```python
from build123d import *
from OCP.BRepAlgoAPI import BRepAlgoAPI_Cut
from OCP.TopTools import TopTools_ListOfShape

# Parameters (mm, degrees)
SKETCH3_R                = 3.65
SKETCH3_R_2              = 2.1
BOSS_EXTRUDE3_DEPTH      = 15
BOSS_EXTRUDE4_DEPTH      = 8
BOSS_EXTRUDE4_DEPTH_BACK = 8
SKETCH7_R                = 2.1
CUT_EXTRUDE1_DEPTH       = 18
FILLET2_START            = -8
FILLET2_DEPTH            = 16
FILLET2_2_ANGLE          = 28.578113
FILLET2_3_ANGLE          = 28.578113


with BuildPart() as part:
    # Sketch3 → Boss-Extrude3 (new body)
    with BuildSketch(Plane(origin=(0, 0, 0), x_dir=(0, 0, -1), z_dir=(1, 0, 0))):
        Circle(SKETCH3_R)
        Circle(SKETCH3_R_2, mode=Mode.SUBTRACT)
    extrude(amount=BOSS_EXTRUDE3_DEPTH)

    # Sketch6 → Boss-Extrude4 (add, two sides: drawn at the far end of the back side and taken through both)
    with BuildSketch(Plane(origin=(0, 0, 0), x_dir=(1, 0, 0), z_dir=(0, 1, 0)).offset(-BOSS_EXTRUDE4_DEPTH_BACK)):
        with BuildLine():
            Line((3.477507, 8.380826), (4.919958, 8.978308))
            ThreePointArc((4.919958, 8.978308), (6.258182, -0.050001), (5.26999, -9.123296))
            Line((5.26999, -9.123296), (3.819467, -8.52247))
            ThreePointArc((3.819467, -8.52247), (4.707866, -0.049391), (3.477507, 8.380826))
        make_face()
    extrude(amount=BOSS_EXTRUDE4_DEPTH + BOSS_EXTRUDE4_DEPTH_BACK)

    # Sketch7 → Cut-Extrude1 (cut)
    with BuildSketch(Plane.ZY):
        with Locations(Location((0, 0, 0), (0, 0, 180))):
            Circle(SKETCH7_R)
    extrude(amount=-CUT_EXTRUDE1_DEPTH, mode=Mode.SUBTRACT)


with BuildPart() as fillet2_tool:
    # Fillet2: read off the stored shape, not the designer's step
    # Fillet2 outline → Fillet2 (new body)
    with BuildSketch(Plane(origin=(0, 0, 0), x_dir=(1, 0, 0), z_dir=(0, 1, 0)).offset(FILLET2_START)):
        with BuildLine():
            ThreePointArc((5.26999, -9.123296), (5.521856, -7.99803), (5.737351, -6.865235))
            ThreePointArc((5.737351, -6.865235), (5.074459, -8.036465), (3.819467, -8.52247))
            Line((3.819467, -8.52247), (5.26999, -9.123296))
        make_face()
        with BuildLine():
            ThreePointArc((3.477507, 8.380826), (4.751128, 7.945976), (5.460847, 6.802514))
            ThreePointArc((5.460847, 6.802514), (5.20744, 7.894646), (4.919958, 8.978308))
            Line((4.919958, 8.978308), (3.477507, 8.380826))
        make_face()
    extrude(amount=FILLET2_DEPTH)


with BuildPart() as part_1:
    add(part.part)

    # Fillet2: cut by fillet2_tool, with a tolerance
    fillet2_stock = TopTools_ListOfShape()
    fillet2_stock.Append(part_1.part.wrapped)
    fillet2_tools = TopTools_ListOfShape()
    fillet2_tools.Append(fillet2_tool.part.wrapped)
    fillet2_cut = BRepAlgoAPI_Cut()
    fillet2_cut.SetArguments(fillet2_stock)
    fillet2_cut.SetTools(fillet2_tools)
    fillet2_cut.SetFuzzyValue(0.00001)
    fillet2_cut.Build()
    add(Compound.cast(fillet2_cut.Shape()).solids(), mode=Mode.REPLACE)


with BuildPart() as fillet2_2_tool:
    # Fillet2 2 outline → Fillet2 2 (revolve)
    with BuildSketch(Plane(origin=(-29.535127, 0, 0.742139), x_dir=(0.9738567621765157, 0, 0.22716295200378364), z_dir=(-0.22716295200378364, 0, 0.9738567621765157))):
        with BuildLine():
            Line((35.8, -8), (35.8, -6.051282))
            ThreePointArc((35.8, -6.051282), (35.365248, -7.296272), (34.25, -8))
            Line((34.25, -8), (35.8, -8))
        make_face()
    revolve(axis=Axis((-29.535127, 0, 0.742139), (0, 1, 0)), revolution_arc=FILLET2_2_ANGLE)


with BuildPart() as part_2:
    add(part_1.part)

    # Fillet2 2: cut by fillet2_2_tool, with a tolerance
    fillet2_2_stock = TopTools_ListOfShape()
    fillet2_2_stock.Append(part_2.part.wrapped)
    fillet2_2_tools = TopTools_ListOfShape()
    fillet2_2_tools.Append(fillet2_2_tool.part.wrapped)
    fillet2_2_cut = BRepAlgoAPI_Cut()
    fillet2_2_cut.SetArguments(fillet2_2_stock)
    fillet2_2_cut.SetTools(fillet2_2_tools)
    fillet2_2_cut.SetFuzzyValue(0.00001)
    fillet2_2_cut.Build()
    add(Compound.cast(fillet2_2_cut.Shape()).solids(), mode=Mode.REPLACE)


with BuildPart() as fillet2_3_tool:
    # Fillet2 3 outline → Fillet2 3 (revolve)
    with BuildSketch(Plane(origin=(-29.535127, 0, 0.742139), x_dir=(0.9738567621765157, 0, 0.22716295200378342), z_dir=(-0.22716295200378342, 0, 0.9738567621765157))):
        with BuildLine():
            ThreePointArc((34.25, 8), (35.365248, 7.296272), (35.8, 6.051282))
            Line((35.8, 6.051282), (35.8, 8))
            Line((35.8, 8), (34.25, 8))
        make_face()
    revolve(axis=Axis((-29.535127, 0, 0.742139), (0, 1, 0)), revolution_arc=FILLET2_3_ANGLE)


with BuildPart() as part_3:
    add(part_2.part)

    # Fillet2 3: cut by fillet2_3_tool, with a tolerance
    fillet2_3_stock = TopTools_ListOfShape()
    fillet2_3_stock.Append(part_3.part.wrapped)
    fillet2_3_tools = TopTools_ListOfShape()
    fillet2_3_tools.Append(fillet2_3_tool.part.wrapped)
    fillet2_3_cut = BRepAlgoAPI_Cut()
    fillet2_3_cut.SetArguments(fillet2_3_stock)
    fillet2_3_cut.SetTools(fillet2_3_tools)
    fillet2_3_cut.SetFuzzyValue(0.00001)
    fillet2_3_cut.Build()
    add(Compound.cast(fillet2_3_cut.Shape()).solids(), mode=Mode.REPLACE)


solid = part_3.part
```
Build history of the part. All positions in model axes, mm. A direction names the side the tool comes from. Coordinates: 2 decimals unless noted, no trailing zeros. Order: outer loops, then holes, each group sorted by start corner. A loop starts at its lowest first (then second) coordinate and runs counter-clockwise, first axis right, second up.
Item 1: Saw through at C-C on y = -2.5. List the corners of the cut face in (x, z), then the cut area to 3 significant figures.
Filled in:
outline: (0, -2.66) - (4.55, -2.66) arc R34.25 cw to (3.48, -8.38) arc R2 ccw to (5.46, -6.8) arc R35.8 ccw to (6.1, -2.66) - (15, -2.66) - (15, 2.66) - (6.21, 2.66) arc R35.8 ccw to (5.74, 6.87) arc R2 ccw to (3.82, 8.52) arc R34.25 cw to (4.66, 2.66) - (0, 2.66) - close
area: 97.0 mm2
Item 2: Drop flat-ended pins along their axis: pin 1 Ø1 at (x, z) = (13.5, 6) entering from -Y; pin 2 Ø1 at (x, z) = (3.5, -2) entering from -Y; pin 3 Ø1.5 at (x, y) = (8, -2) entering from +Z; pin 4 Ø8 at (x, z) = (8.5, -4) entering from -Y. Give the stop position or say it passes through.
Filled in:
pin 1: passes through
pin 2: stops at y = -3.33
pin 3: stops at z = 3.43
pin 4: stops at y = -7.98
Item 3: Saw through at A-A on y = 0. List the corners of the cut face in (x, z).
Filled in:
outline: (0, -3.65) - (4.43, -3.65) arc R34.25 cw to (3.48, -8.38) arc R2 ccw to (5.46, -6.8) arc R35.8 ccw to (5.99, -3.65) - (15, -3.65) - (15, -2.1) - (0, -2.1) - close; (0, 2.1) - (15, 2.1) - (15, 3.65) - (6.15, 3.65) arc R35.8 ccw to (5.74, 6.87) arc R2 ccw to (3.82, 8.52) arc R34.25 cw to (4.59, 3.65) - (0, 3.65) - close
Item 4: Saw through at B-B on x = 11. List the corners of the cut face in (y, z), then the cut area to 3 significant figures.
Filled in:
outline: circle Ø7.3 at (0, 0); hole circle Ø4.2 at (0, 0)
area: 28.0 mm2
Item 5: Saw through at D-D on y = 1.75. List the corners of the cut face in (x, z), then the cut area to 3 significant figures.
Filled in:
outline: (0, -3.2) - (4.49, -3.2) arc R34.25 cw to (3.48, -8.38) arc R2 ccw to (5.46, -6.8) arc R35.8 ccw to (6.05, -3.2) - (15, -3.2) - (15, -1.16) - (0, -1.16) - close; (0, 1.16) - (15, 1.16) - (15, 3.2) - (6.18, 3.2) arc R35.8 ccw to (5.74, 6.87) arc R2 ccw to (3.82, 8.52) arc R34.25 cw to (4.63, 3.2) - (0, 3.2) - close
area: 76.8 mm2
Item 6: Tool access for faces 1 (the cylindrical face through (2.33, 1.1, -3.48)), 2 (the cylindrical face through (6.255, -4.119, -0.078)), 3 (the cylindrical face through (5.089, -0.112, 8.024)): list every direction of +Z, -Z, +X, -X, +Y, -Y with a clear straight run to the whole face (end or side of a thin tool).
Filled in:
face 1: -X
face 2: +X
face 3: +Z, +X, +Y, -Y
Item 7: Drill centre lines: L1, parallel to Z at x = 2, y = 0; L2, parallel to Z at x = 9.25, y = -0.5. Where is each one in solid material? Low to high.
Filled in:
L1: z = -3.65 to -2.1, 2.1 to 3.65
L2: z = -3.62 to -2.04, 2.04 to 3.62
